Could you check a few things on this model? Use its own coordinates, in mm. A direction names the side the tool comes from. Round coordinates to 2 decimals unless told otherwise and drop trailing zeros. Loops run counter-clockwise (first coordinate to the right, second up) from the corner with the lowest first, then second, coordinate; pieces in that order, holes last. Notation, with made-up numbers: M 85,42.5 L 140,42.5 A15 ccw 140,68.5 Z; hole C -16,74.25 d5. An arc over 180 degrees is marked long. Answer in a Markdown table with one row per item.
```python
from build123d import *

# Parameters (mm, degrees)
F1_DEPTH = 9.7
F3_DEPTH = 7.7


with BuildPart() as f1:
    # F0 (on Front) → F1 (new body)
    with BuildSketch(Plane.XZ):
        Polygon((2.5, 8.5), (0, 8.5), (-2.5, 8.5), (-4.45, 5.1225009252), (-4.45, 0), (0, 0), (4.45, 0), (4.45, 5.1225009252), align=None)
    extrude(amount=F1_DEPTH)

    # F2 (on Front) → F3 (cut, through all)
    with BuildSketch(Plane.XZ):
        Polygon((-4.45, 5.1225009252), (-4.45, 3), (-4.1234630536, 3), (-3.2843634225, 2), (0, 2), (0, 8.5), (-2.5, 8.5), align=None)
        Polygon((0, 8.5), (0, 2), (3.2843634225, 2), (4.1234630536, 3), (4.45, 3), (4.45, 5.1225009252), (2.5, 8.5), align=None)
    extrude(amount=F3_DEPTH, mode=Mode.SUBTRACT)

    # F4: F1 across plane


with BuildPart() as f1_1:
    add(f1.part)
    add(f1.part.mirror(Plane.XZ))


solid = f1_1.part
```
1) I want a section at B-B, the plane y = -6. Please give me the cut outline in (x, z), plus the area to 3 significant figures.
Computed:
| item | result |
|---|---|
| outline | M -4.45,0 L 4.45,0 L 4.45,3 L 4.12,3 L 3.28,2 L -3.28,2 L -4.12,3 L -4.45,3 Z |
| area | 19.3 mm² |
2) If we mould it in two halves opening along Y, with no side actions, what happens to faces 1 (the face through (3.698, -0.108, 2.493)), 2 (the face through (0, 9.7, 4)), 3 (the face through (0, 0, 0))? For each: released by +Y, released by -Y, zero draft, split by the parting line, or undercut.
Computed:
| item | result |
|---|---|
| face 1 | undercut |
| face 2 | released by +Y |
| face 3 | zero draft |
3) Which directions (+Z, -Z, +X, -X, +Y, -Y) give clear straight access to the entire face, cutting with the end or side of a thin tool? Please do faces 4 (the face through (-3.71, -0.11, 2.51)), 5 (the face through (0, 9, 8.5)).
Computed:
| item | result |
|---|---|
| face 4 | +Z |
| face 5 | +Z, +X, -X, +Y, -Y |
4) I need wall thicknesses on line 1 (Y direction, x = 1.25, z = 7); line 2 (Z direction, x = -1.75, y = 3.75); line 3 (X direction, y = -7, z = 2.25). Which ranges of each line are inside material? Lowest first, please.
Computed:
| item | result |
|---|---|
| line 1 | y = -9.7 to -7.7, 7.7 to 9.7 |
| line 2 | z = 0 to 2 |
| line 3 | x = -4.45 to -3.49, 3.49 to 4.45 |
5) I want a section at C-C, the plane x = -1.25. Please give me the cut outline in (y, z).
Computed:
| item | result |
|---|---|
| outline | M -9.7,0 L 9.7,0 L 9.7,8.5 L 7.7,8.5 L 7.7,2 L -7.7,2 L -7.7,8.5 L -9.7,8.5 Z |
6) I want a section at D-D, the plane z = 5.5. Please give me the cut outline in (x, y).
Computed:
| item | result |
|---|---|
| outline | M -4.23,-9.7 L 4.23,-9.7 L 4.23,-7.7 L -4.23,-7.7 Z; M -4.23,7.7 L 4.23,7.7 L 4.23,9.7 L -4.23,9.7 Z |
7) I want a section at A-A, the plane z = 7. Please give me the cut outline in (x, y), plus the area to 3 significant figures.
Computed:
| item | result |
|---|---|
| outline | M -3.37,-9.7 L 3.37,-9.7 L 3.37,-7.7 L -3.37,-7.7 Z; M -3.37,7.7 L 3.37,7.7 L 3.37,9.7 L -3.37,9.7 Z |
| area | 26.9 mm² |
8) Will this pin go through, and if not, where does the flat tip stop? P1, Ø1, axis at x = -0.5, y = -3, coming from the +Z side.
Computed:
| item | result |
|---|---|
| P1 | stops at z = 2 |
